Input: part model. Units: mm. Frame: model coordinates. A direction names the side the tool comes from. Round coordinates to 2 decimals unless told otherwise and drop trailing zeros. Loops run counter-clockwise (first coordinate to the right, second up) from the corner with the lowest first, then second, coordinate; pieces in that order, holes last. Notation, with made-up numbers: (7, 78.5) -> (48, 78.5) arc R23 ccw to (48, 98.5) -> close; hole circle Ø9 at (-35, 44). An arc over 180 degrees is marked (long way). Answer in a Markdown table with one row per item. Add a question column.
Q1. Pin query (flat end, axial travel): pin 1 (5.5 mm diameter, centred on x = 4, y = 3.5, fed in from -Z); pin 2 (1.5 mm diameter, centred on x = -4, y = 5.5, fed in from -Z); pin 3 (3.5 mm diameter, centred on x = 14, y = 6.5, fed in from +Z); pin 4 (2 mm diameter, centred on y = 6.5, z = -1.5, fed in from +X). Return the tip coordinate at first contact, or that it passes through.
Q2. Section D-D, the plane y = 1.25. Output: boundary loops of the cut face in (x, z).
Q3. Section A-A, the plane x = 5. Output: boundary loops of the cut face in (y, z), and give its area (3 significant figures).
Q4. Section B-B, the plane z = -0.75. Output: boundary loops of the cut face in (x, y), and give its area (3 significant figures).
Q5. Reachability of faces 1 (the face through (10, 5, -2)), 2 (the face through (7.4, 5.4, -5.6)), 3 (the face through (-3, 5, -3)) from +Z, -Z, +X, -X, +Y, -Y: full face, straight path, thin tool, end or side. Return the list, or none.
Q6. Section C-C, the plane y = 5.25. Output: boundary loops of the cut face in (x, z), and give its area (3 significant figures).
Q7. Ray query, L1, parallel to Y at x = 5, z = -0.8; L2, parallel to Y at x = 5.5, z = -1.5; L3, parallel to X at y = 4.25, z = -4. Return the intervals inside material, ascending. Write a range as from..to.
Q8. Mould query, pull axis Y, two halves, no side actions, for faces 4 (the face through (14, 5, -3)), 5 (the face through (4.17, 4.06, -0.79)), 6 (the face through (5, 0, -4)). Classes: pulls with the +Y half, pulls with the -Y half, needs draft (parallel to the pull), parting line crosses it, or undercut.
```python
from build123d import *

# Parameters (mm, degrees)
BOSS_EXTRU_2_DEPTH      = 9.4
ESQUISSE13_R            = 1
ESQUISSE14_R            = 1.05
ENL_V_MAT_EXTRU_1_DEPTH = 22.590228256
ESQUISSE15_R            = 2.5
ENL_V_MAT_EXTRU_2_DEPTH = 8.4
CONG_2_R                = 0.5
CONG_3_R                = 2


with BuildPart() as part:
    # Esquisse1 → Boss.-Extru.2 (new body)
    with BuildSketch(Plane(origin=(0, 0, 0), x_dir=(1, 0, 0), z_dir=(0, 1, 0))):
        with BuildLine():
            ThreePointArc((-7, 3), (5, 9.422205102), (17, 3))
            Line((17, 3), (10, 3))
            Line((10, 3), (10, 0))
            Line((10, 0), (0, 0))
            Line((0, 0), (0, 3))
            Line((0, 3), (-7, 3))
        make_face()
    extrude(amount=BOSS_EXTRU_2_DEPTH)

    # Esquisse13 → Enlèvement de matière-Révolution4 (revolve, cut)
    with BuildSketch(Plane.XY.offset(5)):
        with Locations((-10, 4.7)):
            Circle(ESQUISSE13_R)
    revolve(axis=Axis((5, 9.4, 5), (0, -1, 0)), mode=Mode.SUBTRACT)

    # Esquisse14 → Enlèv. mat.-Extru.1 (cut, through all)
    with BuildSketch(Plane.XY):
        with Locations((5, 4.7)):
            Circle(ESQUISSE14_R)
    extrude(amount=-ENL_V_MAT_EXTRU_1_DEPTH, mode=Mode.SUBTRACT)

    # Esquisse15 → Enlèv. mat.-Extru.2 (cut)
    with BuildSketch(Plane.XY.offset(-10)):
        with Locations(Location((5, 4.7, 0), (0, 0, 199.054827186))):
            Circle(ESQUISSE15_R)
    extrude(amount=ENL_V_MAT_EXTRU_2_DEPTH, mode=Mode.SUBTRACT)

    # Congé2
    cong_2_edges = [part.edges().sort_by_distance(p)[0] for p in [
        (10, 4.7, 0),
        (0, 4.7, 0),
        (5, 9.4, 0),
        (5, 0, 0),
    ]]
    fillet(cong_2_edges, radius=CONG_2_R)

    # Congé3
    cong_3_edges = [part.edges().sort_by_distance(p)[0] for p in [
        (5, 0, -9.422205102),
        (5, 9.4, -9.422205102),
    ]]
    fillet(cong_3_edges, radius=CONG_3_R)


solid = part.part
```
Answer block:
| question | item | result |
|---|---|---|
| 1 | pin 1 | z = -9.42 |
| 1 | pin 2 | z = -6.83 |
| 1 | pin 3 | z = -3 |
| 1 | pin 4 | x = 10 |
| 2 | outline | (-6.82, -3) arc R14.28 ccw to (16.82, -3) -> (10, -3) -> (10, -0.5) arc R0.5 ccw to (9.5, 0) -> (0.5, 0) arc R0.5 ccw to (0, -0.5) -> (0, -3) -> close |
| 3 | outline | (0, -7.42) arc R2 ccw to (2, -9.42) -> (2.2, -9.42) -> (2.2, -1.6) -> (3.65, -1.6) -> (3.65, 0) -> (0.5, 0) arc R0.5 ccw to (0, -0.5) -> close; (5.75, -1.6) -> (7.2, -1.6) -> (7.2, -9.42) -> (7.4, -9.42) arc R2 ccw to (9.4, -7.42) -> (9.4, -0.5) arc R0.5 ccw to (8.9, 0) -> (5.75, 0) -> close |
| 3 | area | 44.3 mm^2 |
| 4 | outline | (0, 0) -> (10, 0) -> (10, 9.4) -> (0, 9.4) -> close; hole circle Ø2.1 at (5, 4.7) |
| 4 | area | 90.5 mm^2 |
| 5 | face 1 | +Z, +X, +Y, -Y |
| 5 | face 2 | -Z |
| 5 | face 3 | +Z, -X, +Y, -Y |
| 6 | outline | (-6.69, -3) arc R14.16 ccw to (2.56, -8.95) -> (2.56, -1.6) -> (4.11, -1.6) -> (4.11, 0) -> (0.5, 0) arc R0.5 ccw to (0, -0.5) -> (0, -3) -> close; (5.89, -1.6) -> (7.44, -1.6) -> (7.44, -8.95) arc R14.16 ccw to (16.69, -3) -> (10, -3) -> (10, -0.5) arc R0.5 ccw to (9.5, 0) -> (5.89, 0) -> close |
| 6 | area | 91.7 mm^2 |
| 7 | L1 | 0..3.65, 5.75..9.4 |
| 7 | L2 | 0..3.78, 5.62..9.4 |
| 7 | L3 | -5.86..2.54, 7.46..15.86 |
| 8 | face 4 | needs draft |
| 8 | face 5 | undercut |
| 8 | face 6 | pulls with the -Y half |
